from build123d import *

# Parameters (mm, degrees)
BOSS_EXTRUDE1_DEPTH       = 150
CUT_EXTRUDE1_REACH        = 36
SKETCH2_R                 = 12.5
CUT_EXTRUDE2_REACH        = 36
SKETCH3_R                 = 2.1
F_3_0MM_DOWEL_HOLE1_D     = 3
F_3_0MM_DOWEL_HOLE1_DEPTH = 2
F_3_0MM_DOWEL_HOLE2_D     = 3
F_3_0MM_DOWEL_HOLE2_DEPTH = 2.001


with BuildPart() as part:
    # Sketch1 → Boss-Extrude1 (new body)
    with BuildSketch(Plane.XY):
        Polygon((-77, 17), (77, 17), (77, -15), (107, -15), (107, -17), (75, -17), (75, 15), (-75, 15), (-75, -17), (-107, -17), (-107, -15), (-77, -15), align=None)
    extrude(amount=BOSS_EXTRUDE1_DEPTH)

    # Sketch2 → Cut-Extrude1 (cut, up to next)
    with BuildSketch(Plane(origin=(0, 17, 0), x_dir=(1, 0, 0), z_dir=(0, 1, 0)), mode=Mode.PRIVATE) as cut_extrude1_sk1:
        with Locations((8, -75)):
            Circle(SKETCH2_R)
    cut_extrude1_tool1 = extrude(cut_extrude1_sk1.sketch, amount=-CUT_EXTRUDE1_REACH, mode=Mode.PRIVATE) & part.part
    add(cut_extrude1_tool1.solids().sort_by_distance((8, 17, 75))[0], mode=Mode.SUBTRACT)

    # Sketch3 → Cut-Extrude2 (cut, up to next)
    with BuildSketch(Plane(origin=(0, 17, 0), x_dir=(1, 0, 0), z_dir=(0, 1, 0)), mode=Mode.PRIVATE) as cut_extrude2_sk1:
        with Locations((8, -57.5)):
            Circle(SKETCH3_R)
    cut_extrude2_tool1 = extrude(cut_extrude2_sk1.sketch, amount=-CUT_EXTRUDE2_REACH, mode=Mode.PRIVATE) & part.part
    add(cut_extrude2_tool1.solids().sort_by_distance((8, 17, 57.5))[0], mode=Mode.SUBTRACT)
    # Sketch3 → Cut-Extrude2 (cut, up to next)
    with BuildSketch(Plane(origin=(0, 17, 0), x_dir=(1, 0, 0), z_dir=(0, 1, 0)), mode=Mode.PRIVATE) as cut_extrude2_sk2:
        with Locations((8, -92.5)):
            Circle(SKETCH3_R)
    cut_extrude2_tool2 = extrude(cut_extrude2_sk2.sketch, amount=-CUT_EXTRUDE2_REACH, mode=Mode.PRIVATE) & part.part
    add(cut_extrude2_tool2.solids().sort_by_distance((8, 17, 92.5))[0], mode=Mode.SUBTRACT)

    # Ø3.0mm Dowel Hole1
    with Locations(Plane(origin=(0, 15, 0), x_dir=(-1, 0, 0), z_dir=(0, -1, 0))):
        with Locations((58.5, -111.5), (58.5, -96.5), (37.5, -131.5), (22.5, -131.5), (-22.5, -131.5), (-37.5, -131.5), (-58.5, -111.5), (-58.5, -96.5), (-58.5, -53.5), (-58.5, -38.5), (-37.5, -18.5), (-22.5, -18.5), (22.5, -18.5), (37.5, -18.5), (58.5, -53.5), (58.5, -38.5)):
            Hole(F_3_0MM_DOWEL_HOLE1_D / 2, depth=F_3_0MM_DOWEL_HOLE1_DEPTH)

    # Ø3.0mm Dowel Hole2
    with Locations(Plane.ZY.offset(-75)):
        with Locations((38.5, -3.5), (53.5, -3.5), (96.5, -3.5), (111.5, -3.5)):
            f_3_0mm_dowel_hole2 = Hole(F_3_0MM_DOWEL_HOLE2_D / 2, depth=F_3_0MM_DOWEL_HOLE2_DEPTH)

    # Mirror1: Ø3.0mm Dowel Hole2 across plane
    add(f_3_0mm_dowel_hole2.mirror(Plane(origin=(0, 0, 0), x_dir=(0, 0, 1), z_dir=(1, 0, 0))), mode=Mode.SUBTRACT)


solid = part.part
Can you work these out from the model? Positions are in its coordinate system, mm. A direction names the side the tool comes from. Round coordinates to 2 decimals unless told otherwise and drop trailing zeros. Write each loop counter-clockwise with the first axis right and the second up, starting at its lowest first coordinate (ties: lowest second). Pieces come first, ordered by that corner, then holes. Notation, with made-up numbers: (70, 33.5) -> (74, 33.5) arc R24 ccw to (74, 43.5) -> close; hole circle Ø6 at (3.25, 3.5). An arc over 180 degrees is marked (long way). Use one line per item in the form item = value. Start each with the question number.
Q1. Imagine slicing it at A-A (y = 3). Please give me the cut outline in (x, z).
Q2. Which directions (+Z, -Z, +X, -X, +Y, -Y) give clear straight access to the entire face, cutting with the end or side of a thin tool? Please do faces 1 (the face through (-91, -17, 74)), 2 (the face through (-77, 1, 74)), 3 (the face through (-16, 15, 74)), 4 (the face through (6.334, 16.014, 58.778)), 5 (the face through (77, 1, 74)).
Q3. I'm going to push flat-ended pins straight in: P1, Ø6, axis at y = -8.5, z = 15.5, coming from the -X side; P2, Ø3.5, axis at x = 58.5, z = 96.5, coming from the -Y side; P3, Ø10, axis at y = 0.5, z = 33.5, coming from the +X side. Where does each tip first touch, or does it pass through?
Q4. If I drill on probe 1 along X at (y, z) = (15.7, 18.5); probe 2 along Z at (x, y) = (8, 16.45); probe 3 along X at (y, z) = (16.05, 75), over which ranges is the centre line in solid material (lowest first)? Write a range as [from, to].
Q5. Imagine slicing it at B-B (x = -63). Please give me the cut outline in (y, z).
Q6. We'd pull the mould along Z, two halves only. Please class faces 6 (the face through (0.5, 15.2, 0)), 7 (the face through (91, -17, 74)), 8 (the face through (0.5, 15.2, 150)), 9 (the face through (6.373, 16.014, 62.606)): +Z half, -Z half, draft (parallel to the pull), parting line (faces both ways), or undercut.
Worked out:
q1.outline = (-77, 0) -> (-75, 0) -> (-75, 150) -> (-77, 150) -> close; (75, 0) -> (77, 0) -> (77, 150) -> (75, 150) -> close
q2.face_1 = +Z, -Z, +X, -X, -Y
q2.face_2 = +Z, -Z, -X, +Y
q2.face_3 = +Z, -Z, -Y
q2.face_4 = +Y, -Y
q2.face_5 = +Z, -Z, +X, +Y
q3.P1 = -77
q3.P2 = 15
q3.P3 = 77
q4.probe_1 = [-77, -39], [-36, -24], [-21, 21], [24, 36], [39, 77]
q4.probe_2 = [0, 55.4], [59.6, 62.5], [87.5, 90.4], [94.6, 150]
q4.probe_3 = [-77, -4.5], [20.5, 77]
q5.outline = (15, 0) -> (17, 0) -> (17, 150) -> (15, 150) -> close
q6.face_6 = -Z half
q6.face_7 = draft
q6.face_8 = +Z half
q6.face_9 = undercut
